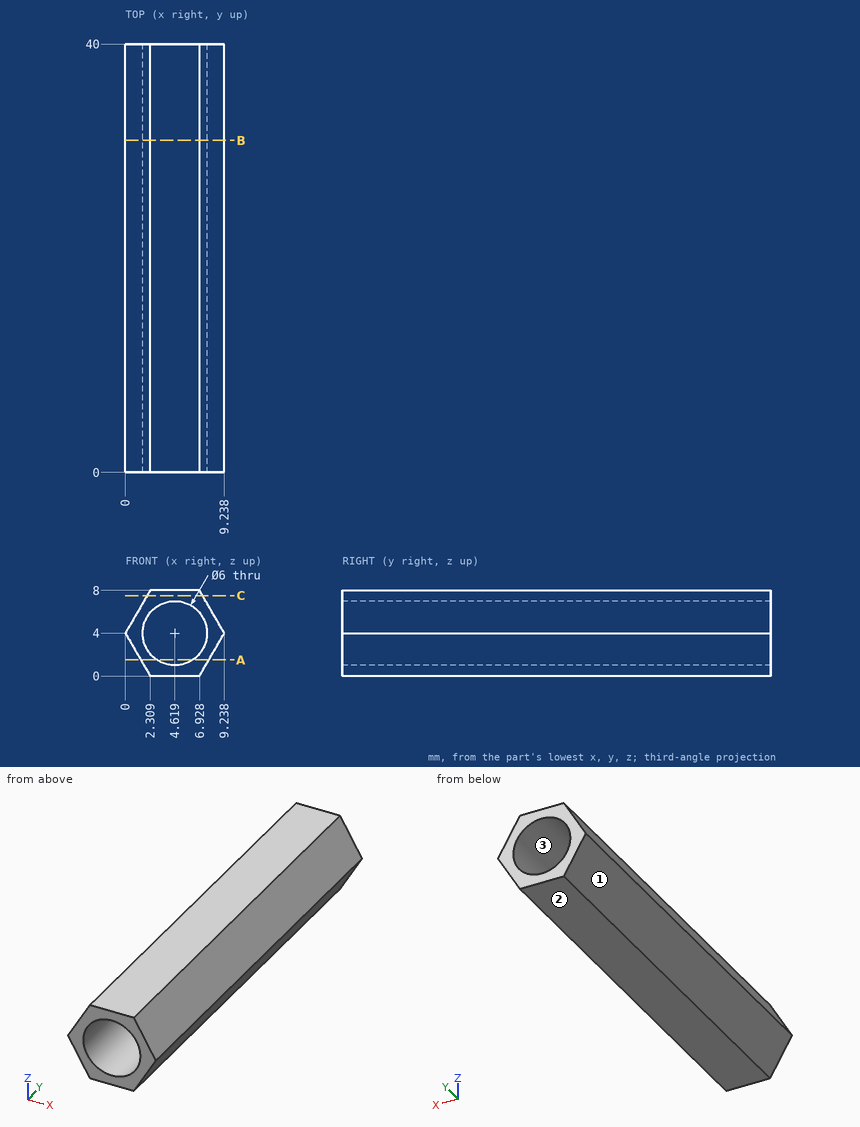
The drawing under review shows one solid part. Ordinate dimensions are in mm from its lowest x, y, z. Round coordinates to 2 decimals unless told otherwise and drop trailing zeros. Write each loop counter-clockwise with the first axis right and the second up, starting at its lowest first coordinate (ties: lowest second). Pieces come first, ordered by that corner, then holes.
(1) Mouldability with a two-part tool opening along X and no side actions: class the marked faces 1, 2 and 3 as +X half, -X half, draft (parallel to the pull), parting line (faces both ways), or undercut.
(2) We need section B-B on y = 31. Give the boundary of the cut face in (x, z).
(3) Insertion check: pin 1 (4 mm diameter, centred on y = 27.5, z = 5, fed in from -X). The pin has a flat end and moves straight along its axis. Give the tip position at first contact, or say it passes through.
(4) Wall thickness on L1, parallel to Z at x = 4.5, y = 9.5; L2, parallel to Z at x = 5.5, y = 8; L3, parallel to X at y = 30, z = 2.5 (1 decimal): over which ranges is each line inside the solid? List them lowest first.
(5) We need section A-A on z = 1.5. Give the boundary of the cut face in (x, y) (1 decimal).
(6) We need section C-C on z = 7.5. Give the boundary of the cut face in (x, y), and give its area (3 significant figures).
Findings below:
1. face 1: -X half
1. face 2: draft
1. face 3: undercut
2. outline: (0, 4) - (2.31, 0) - (6.93, 0) - (9.24, 4) - (6.93, 8) - (2.31, 8) - close; hole circle Ø6 at (4.62, 4)
3. pin 1: stops at x = 0
4. L1: z = 0 to 1, 7 to 8
4. L2: z = 0 to 1.13, 6.87 to 8
4. L3: x = 0.9 to 2, 7.2 to 8.4
5. outline: (1.4, 0) - (3, 0) - (3, 40) - (1.4, 40) - close; (6.3, 0) - (7.8, 0) - (7.8, 40) - (6.3, 40) - close
6. outline: (2.02, 0) - (7.22, 0) - (7.22, 40) - (2.02, 40) - close
6. area: 208 mm2
